Read the model definition and answer for the solid it produces. Units are mm, in the model's axes. A direction names the side the tool comes from. Coordinates: 2 decimals unless noted, no trailing zeros. Write each loop counter-clockwise with the first axis right and the second up, starting at its lowest first coordinate (ties: lowest second). Pieces come first, ordered by that corner, then holes.
(1) Find the intervals of material crossed by probe 1 along Z at (x, y) = (-76, 3.5); probe 2 along X at (y, z) = (2.25, 3.5); probe 3 along X at (y, z) = (5.25, -2), in increasing order.
(2) The mould has two halves that part along Y. Classify faces 4 (the cylindrical face through (77.85, 9.99, 28.04)), 5 (the flat face through (82, 7, 30.5)), 6 (the cylindrical face through (-82, 8, 0)): +Y half, -Y half, draft (parallel to the pull), parting line (faces both ways), or undercut.
(3) Given pin 1 (5 mm diameter, centred on x = 79, y = 9.5, fed in from -Z); pin 2 (1 mm diameter, centred on x = -63, z = -17, fed in from +Y); pin 3 (4 mm diameter, centred on y = 11.5, z = -0.5, fed in from +X); pin 4 (2.5 mm diameter, centred on y = 1, z = 17, fed in from +X), each flat-ended and moving along its own axis, determine where each tip first touches the part or whether it passes through.
(4) Section B-B on x = -22 is taken. Write down the section's boundary in (y, z), then the cut area to 3 significant figures.
(5) Section A-A on x = 26 is taken. Write down the section's boundary in (y, z).
(6) Which of the six approach directions +Z, -Z, +X, -X, +Y, -Y give full straight-line access (tool end or side, diameter ignored) to faces 1 (the flat face through (-52, 1, 22.5)), 2 (the flat face through (-82, 7, 25.5)), 3 (the cylindrical face through (-64.117, 2.014, 1.197))?
from build123d import *

# Parameters (mm, degrees)
SKIZZE1_W                                  = 180
SKIZZE1_H                                  = 65
AUFSATZ_LINEAR_AUSTRAGEN1_DEPTH            = 3
SKIZZE2_W                                  = 25
SKIZZE2_H                                  = 15
SCHNITT_LINEAR_AUSTRAGEN1_DEPTH            = 3
SKIZZE3_W                                  = 5
SKIZZE3_H                                  = 7
AUFSATZ_LINEAR_AUSTRAGEN2_DEPTH            = 6
F_4_0_4_DURCHMESSER_BOHRUNG1_D             = 4
SCHNITT_LINEAR_AUSTRAGEN4_DEPTH            = 112.382224794
SKIZZE7_W                                  = 10
SKIZZE7_H                                  = 5
AUFSATZ_LINEAR_AUSTRAGEN3_DEPTH            = 10
SPIEGELN1_AT_THE_SECOND_PLANE_COPY_1_SKE_W = 10
SPIEGELN1_AT_THE_SECOND_PLANE_COPY_1_SKE_H = 5
SPIEGELN1_AT_THE_SECOND_PLANE_COPY_1_DEPTH = 10
VERRUNDUNG2_R                              = 10
F_4_0_4_DURCHMESSER_BOHRUNG3_D             = 4
F_4_0_4_DURCHMESSER_BOHRUNG3_DEPTH         = 5
F_4_0_4_DURCHMESSER_BOHRUNG4_D             = 4
F_4_0_4_DURCHMESSER_BOHRUNG4_DEPTH         = 5
SKIZZE14_R                                 = 3.5
SKIZZE14_R_2                               = 6.75
SKIZZE14_R_3                               = 4
SCHNITT_LINEAR_AUSTRAGEN5_DEPTH            = 92.549167118
SKIZZE17_R                                 = 1.4
SCHNITT_LINEAR_AUSTRAGEN6_DEPTH            = 2


with BuildPart() as part:
    # Skizze1 → Aufsatz-Linear austragen1 (new body)
    with BuildSketch(Plane(origin=(0, 0, 0), x_dir=(1, 0, 0), z_dir=(0, 1, 0))):
        Rectangle(SKIZZE1_W, SKIZZE1_H)
    extrude(amount=AUFSATZ_LINEAR_AUSTRAGEN1_DEPTH)

    # Skizze2 → Schnitt-Linear austragen1 (cut)
    with BuildSketch(Plane(origin=(0, 0, 0), x_dir=(-1, 0, 0), z_dir=(0, -1, 0))):
        with Locations((52.5, -15)):
            Rectangle(SKIZZE2_W, SKIZZE2_H)
    extrude(amount=-SCHNITT_LINEAR_AUSTRAGEN1_DEPTH, mode=Mode.SUBTRACT)

    # Skizze3 → Aufsatz-Linear austragen2 (add)
    with BuildSketch(Plane(origin=(0, 3, 0), x_dir=(1, 0, 0), z_dir=(0, 1, 0))):
        with Locations((-82.5, 0)):
            Rectangle(SKIZZE3_W, SKIZZE3_H)
        with Locations((82.5, 0)):
            Rectangle(SKIZZE3_W, SKIZZE3_H)
    extrude(amount=AUFSATZ_LINEAR_AUSTRAGEN2_DEPTH)

    # Ø4.0 (4) Durchmesser Bohrung1 (through all)
    with Locations(Plane.ZY.offset(85)):
        with Locations((0, 6)):
            Hole(F_4_0_4_DURCHMESSER_BOHRUNG1_D / 2)

    # Skizze4 → Schnitt-Linear austragen4 (cut, through all)
    with BuildSketch(Plane.XY.offset(32.5)):
        with BuildLine():
            Line((-80, 0), (-90, 0))
            Line((-90, 0), (-90, 3))
            Line((-90, 3), (-85, 3))
            Line((-85, 3), (-85, 1.339745962))
            ThreePointArc((-85, 1.339745962), (-82.588190451, 0.340741737), (-80, 0))
        make_face()
        with BuildLine():
            Line((80, 0), (90, 0))
            Line((90, 0), (90, 3))
            Line((90, 3), (85, 3))
            Line((85, 3), (85, 1.339745962))
            ThreePointArc((85, 1.339745962), (82.588190451, 0.340741737), (80, 0))
        make_face()
    extrude(amount=-SCHNITT_LINEAR_AUSTRAGEN4_DEPTH, mode=Mode.SUBTRACT)

    # Skizze7 → Aufsatz-Linear austragen3 (add)
    with BuildSketch(Plane(origin=(0, 3, 0), x_dir=(1, 0, 0), z_dir=(0, 1, 0))):
        with Locations((-80, 28)):
            Rectangle(SKIZZE7_W, SKIZZE7_H)
    aufsatz_linear_austragen3 = extrude(amount=AUFSATZ_LINEAR_AUSTRAGEN3_DEPTH)

    # Spiegeln1: Aufsatz-Linear austragen3 across plane
    add(aufsatz_linear_austragen3.mirror(Plane(origin=(0, 0, 0), x_dir=(0, 0, 1), z_dir=(1, 0, 0))))

    # Spiegeln1 at the second plane: Aufsatz-Linear austragen3 across plane
    add(aufsatz_linear_austragen3.mirror(Plane.XY))

    # Spiegeln1 at the second plane copy 1 ske → Spiegeln1 at the second plane copy 1 (add)
    with BuildSketch(Plane(origin=(0, 3, 0), x_dir=(-1, 0, 0), z_dir=(0, 1, 0))):
        with Locations((-80, 28)):
            Rectangle(SPIEGELN1_AT_THE_SECOND_PLANE_COPY_1_SKE_W, SPIEGELN1_AT_THE_SECOND_PLANE_COPY_1_SKE_H)
    extrude(amount=SPIEGELN1_AT_THE_SECOND_PLANE_COPY_1_DEPTH)

    # Verrundung2
    verrundung2_edges = [part.edges().sort_by_distance(p)[0] for p in [
        (-75, 13, -28),
        (-75, 13, 28),
        (75, 13, -28),
        (75, 13, 28),
    ]]
    fillet(verrundung2_edges, radius=VERRUNDUNG2_R - 0.0001)  # a hair under: the kernel refuses the full size

    # Ø4.0 (4) Durchmesser Bohrung3
    with Locations(Plane(origin=(0, 0, -30.5), x_dir=(-1, 0, 0), z_dir=(0, 0, -1))):
        with Locations((-80, 8), (80, 8)):
            Hole(F_4_0_4_DURCHMESSER_BOHRUNG3_D / 2, depth=F_4_0_4_DURCHMESSER_BOHRUNG3_DEPTH)

    # Ø4.0 (4) Durchmesser Bohrung4
    with Locations(Plane.XY.offset(30.5)):
        with Locations((-80, 8), (80, 8)):
            Hole(F_4_0_4_DURCHMESSER_BOHRUNG4_D / 2, depth=F_4_0_4_DURCHMESSER_BOHRUNG4_DEPTH)

    # Skizze14 → Schnitt-Linear austragen5 (cut, through all)
    with BuildSketch(Plane(origin=(0, 3, 0), x_dir=(1, 0, 0), z_dir=(0, 1, 0))):
        with Locations(Location((26, -2.5, 0), (0, 0, 270))):
            Circle(SKIZZE14_R)
        with Locations(Location((65, -2.5, 0), (0, 0, 270))):
            Circle(SKIZZE14_R_2)
        with Locations(Location((-22, -22.5, 0), (0, 0, 270))):
            Circle(SKIZZE14_R_3)
    extrude(amount=-SCHNITT_LINEAR_AUSTRAGEN5_DEPTH, mode=Mode.SUBTRACT)

    # Skizze17 → Schnitt-Linear austragen6 (cut)
    with BuildSketch(Plane(origin=(0, 3, 0), x_dir=(1, 0, 0), z_dir=(0, 1, 0))):
        with Locations(Location((-62.75, -1.5, 0), (0, 0, 270))):
            Circle(SKIZZE17_R)
        with Locations(Location((-42.25, -1.5, 0), (0, 0, 270))):
            Circle(SKIZZE17_R)
    extrude(amount=-SCHNITT_LINEAR_AUSTRAGEN6_DEPTH, mode=Mode.SUBTRACT)


solid = part.part
Response:
1. probe 1: z = -30.5 to -25.5, 25.5 to 30.5
1. probe 2: x = -85 to 22.65, 29.35 to 58.32, 71.68 to 85
1. probe 3: x = -85 to -80, 80 to 85
2. face 4: +Y half
2. face 5: draft
2. face 6: undercut
3. pin 1: stops at z = -30.5
3. pin 2: stops at y = 3
3. pin 3: passes through
3. pin 4: stops at x = 85
4. outline: (0, -32.5) - (3, -32.5) - (3, 18.5) - (0, 18.5) - close; (0, 26.5) - (3, 26.5) - (3, 32.5) - (0, 32.5) - close
4. area: 171 mm2
5. outline: (0, -32.5) - (3, -32.5) - (3, -1) - (0, -1) - close; (0, 6) - (3, 6) - (3, 32.5) - (0, 32.5) - close
6. face 1: +Y, -Y
6. face 2: +X, -X, +Y
6. face 3: +Y
